from build123d import *

# Parameters (mm, degrees)
F0_R     = 92.075
F0_R_2   = 20.75
F1_DEPTH = 25.4
F2_R     = 10.125
F2_R_2   = 10.25
F2_R_3   = 10
F3_DEPTH = 25.4
F5_D     = 13.49248
F6_SIZE  = 3.175
F7_SIZE  = 0.762


with BuildPart() as f1:
    # F0 (on Front) → F1 (new body)
    with BuildSketch(Plane.XZ):
        Circle(F0_R)
        Circle(F0_R_2, mode=Mode.SUBTRACT)
    extrude(amount=-F1_DEPTH)

    # F2 (on face) → F3 (cut)
    with BuildSketch(Plane.XZ):
        with Locations((-57.1871926221, 20.125)):
            Circle(F2_R)
        with Locations((-20.25, 57.010415715)):
            Circle(F2_R_2)
        with Locations((56.9371926221, -20.4780090433)):
            Circle(F2_R)
        with Locations((20, -57.3634247583)):
            Circle(F2_R_3)
    extrude(amount=-F3_DEPTH, mode=Mode.SUBTRACT)

    # F5 (through all)
    with Locations(Plane.XZ):
        with Locations((-35.9210244843, 35.9210244843), (35.9210244843, 35.9210244843), (35.9210244843, -35.9210244843), (-35.9210244843, -35.9210244843)):
            Hole(F5_D / 2)

    # F6
    f6_edges = [f1.edges().sort_by_distance(p)[0] for p in [
        (92.075, 12.7, 0),
        (-92.075, 0, 0),
        (-92.075, 25.4, 0),
    ]]
    chamfer(f6_edges, length=F6_SIZE)

    # F7
    f7_edges = [f1.edges().sort_by_distance(p)[0] for p in [
        (-47.062193, 12.7, 20.125),
        (-67.312193, 0, 20.125),
        (-67.312193, 25.4, 20.125),
        (-10, 12.7, 57.010416),
        (-30.5, 0, 57.010416),
        (-30.5, 25.4, 57.010416),
        (67.062193, 12.7, -20.478009),
        (46.812193, 0, -20.478009),
        (46.812193, 25.4, -20.478009),
        (30, 12.7, -57.363425),
        (10, 0, -57.363425),
        (10, 25.4, -57.363425),
        (-42.667264, 0, -35.921024),
        (29.174784, 0, -35.921024),
        (-42.667264, 0, 35.921024),
        (29.174784, 0, 35.921024),
        (-42.667264, 25.4, -35.921024),
        (29.174784, 25.4, -35.921024),
        (-42.667264, 25.4, 35.921024),
        (29.174784, 25.4, 35.921024),
    ]]
    chamfer(f7_edges, length=F7_SIZE)


solid = f1.part
Source: CAD feature listing. Evaluate the final solid. Frame: model axes, mm. Coordinates: 2 decimals unless noted, no trailing zeros. Order: outer loops, then holes, each group sorted by start corner. A loop starts at its lowest first (then second) coordinate and runs counter-clockwise, first axis right, second up.
Item 1: Pull-direction query (X, two-part tool) for faces 1 (the face through (-21, 0, 1)), 2 (the face through (40.893, 12.867, 40.48)); classes: pulls with the +X half, pulls with the -X half, needs draft (parallel to the pull), parting line crosses it, or undercut.
Output values:
face 1: needs draft
face 2: undercut
Item 2: Cut plane C-C (y = 11.5). Count the separate pieces of the cut face and the enclosed holes in it, plus the area to 3 significant figures.
Output values:
separate pieces: 1
enclosed holes: 9
area: 23,400 mm2
Item 3: Material intervals for line 1 (X direction, y = 16.5, z = -17); line 2 (X direction, y = 13.75, z = 37); line 3 (X direction, y = 3.25, z = 58), sorted ascending.
Output values:
line 1: x = -90.49 to -11.9, 11.9 to 47.43, 66.45 to 90.49
line 2: x = -84.31 to -42.58, -29.26 to 29.26, 42.58 to 84.31
line 3: x = -71.51 to -30.45, -10.05 to 71.51
Item 4: Cut plane B-B (z = 0). Return loops of the section in (x, y) (3 decimals), plus the area to 3 significant figures.
Output values:
outline: (-92.075, 3.175) - (-88.9, 0) - (-20.75, 0) - (-20.75, 25.4) - (-88.9, 25.4) - (-92.075, 22.225) - close; (20.75, 0) - (88.9, 0) - (92.075, 3.175) - (92.075, 22.225) - (88.9, 25.4) - (20.75, 25.4) - close
area: 3,600 mm2
Item 5: Cut plane A-A (x = 0). Return loops of the section in (y, z) (3 decimals), plus the area to 3 significant figures.
Output values:
outline: (0, -88.9) - (3.175, -92.075) - (22.225, -92.075) - (25.4, -88.9) - (25.4, -20.75) - (0, -20.75) - close; (0, 20.75) - (25.4, 20.75) - (25.4, 88.9) - (22.225, 92.075) - (3.175, 92.075) - (0, 88.9) - close
area: 3,600 mm2
Item 6: First-contact query: P1, Ø5, axis at x = 15.5, y = 10, coming from the +Z side; P2, Ø1.5, axis at y = 18, z = 23.5, coming from the +X side; P3, Ø18, axis at x = -57.19, z = 20.12, coming from the -Y side; P4, Ø12, axis at y = 8, z = 27.5, coming from the +X side. Flat tips, straight axial feed; report the tip coordinate or a pass-through.
Output values:
P1: stops at z = 91.15
P2: stops at x = 89.22
P3: passes through
P4: stops at x = 89.53
